Geometry: final body of the model. Coordinates: model frame, mm. Face numbers are marked on the shaded views. Give positions to 0.01 mm unless a question says otherwise; leave off trailing zeros. Loops run counter-clockwise (first coordinate to the right, second up) from the corner with the lowest first, then second, coordinate; pieces in that order, holes last.
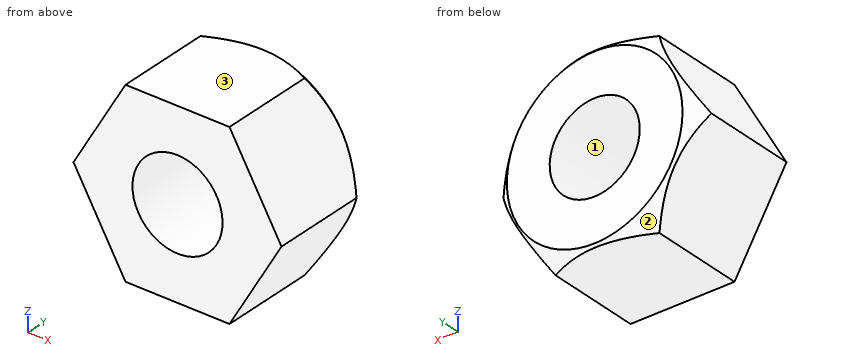
from build123d import *

# Parameters (mm, degrees)
SKETCH_1_R      = 6
EXTRUDE_1_DEPTH = 14.8


with BuildPart() as part:
    # 草图1 → 凸台-拉伸1 (new body)
    with BuildSketch(Plane(origin=(0, 0, 0), x_dir=(1, 0, 0), z_dir=(0, 1, 0))):
        Polygon((-6.92820323, 12), (-13.856406461, 0), (-6.92820323, -12), (6.92820323, -12), (13.856406461, 0), (6.92820323, 12), align=None)
        with Locations(Location((0, 0, 0), (0, 0, 270))):
            Circle(SKETCH_1_R, mode=Mode.SUBTRACT)
    extrude(amount=EXTRUDE_1_DEPTH)

    # 草图2 → 切除-旋转1 (revolve, cut)
    with BuildSketch(Plane.XY, mode=Mode.PRIVATE) as cut_revolve_1_sk:
        Polygon((9.5, 17), (15, 11.5), (15, 17), align=None)
    revolve(cut_revolve_1_sk.sketch.rotate(Axis((0, 17.647957279, 0), (0, -1, 0)), 300.00000004), axis=Axis((0, 17.647957279, 0), (0, -1, 0)), mode=Mode.SUBTRACT)


solid = part.part
Item 1: Pin query (flat end, axial travel): pin 1 (6 mm diameter, centred on y = 7, z = 5.5, fed in from -X); pin 2 (2 mm diameter, centred on x = -8.5, y = 10, fed in from -Z); pin 3 (8 mm diameter, centred on y = 2.5, z = 8.5, fed in from +X). Return the tip coordinate at first contact, or that it passes through.
Values follow:
pin 1: stops at x = -12.41
pin 2: stops at z = -11.01
pin 3: stops at x = 11.26
Item 2: Section query A-A on x = 0. Return loops of the section in (y, z), plus the area to 3 significant figures.
Values follow:
outline: (0, -12) - (14.5, -12) - (14.8, -11.7) - (14.8, -6) - (0, -6) - close; (0, 6) - (14.8, 6) - (14.8, 11.7) - (14.5, 12) - (0, 12) - close
area: 178 mm2
Item 3: Ray query, probe 1 along Z at (x, y) = (0.5, 12.75); probe 2 along X at (y, z) = (2.5, -1); probe 3 along X at (y, z) = (1.5, 1.5). Return the intervals inside material, ascending.
Values follow:
probe 1: z = -12 to -5.98, 5.98 to 12
probe 2: x = -13.28 to -5.92, 5.92 to 13.28
probe 3: x = -12.99 to -5.81, 5.81 to 12.99
Item 4: Draft query along X for the marked faces 1, 2 and 3. Return one class per face: +X half, -X half, draft (parallel to the pull), parting line (faces both ways), or undercut.
Values follow:
face 1: undercut
face 2: parting line
face 3: draft
Item 5: Section query B-B on y = 12. Return loops of the section in (x, z), plus the area to 3 significant figures.
Values follow:
outline: (-13.86, 0) - (-6.93, -12) - (6.93, -12) - (13.86, 0) - (6.93, 12) - (-6.93, 12) - close; hole circle Ø12 at (0, 0)
area: 386 mm2
